from build123d import *

# Parameters (mm, degrees)
F0_R         = 10.3
F1_DEPTH     = 9
F3_R         = 3.1
F4_DEPTH     = 9.001
F6_DEPTH     = 1.8
F7_T4_ANGLE  = 359.64
F7_S5_R      = 3.1
F7_T6_DEPTH  = 5
F7_T10_ANGLE = 359.64
F7_S11_R     = 3.1
F7_T12_DEPTH = 5
F7_T16_ANGLE = 359.64
F7_S17_R     = 3.1
F7_T18_DEPTH = 5
F9_R         = 12.75
F10_DEPTH    = 25
F11_R        = 3.1
F12_DEPTH    = 34.0010001
F13_R        = 12.75
F13_R_2      = 11.35
F14_DEPTH    = 20
F16_DEPTH    = 5
F17_R        = 10.3
F18_DEPTH    = 34.0010001
F20_START    = -5
F20_DEPTH    = 5
F21_R        = 10.3
F21_R_2      = 9.3
F22_DEPTH    = 8
F23_R        = 0.99999


# Not quite as in the source:
# - a fillet or chamfer that OpenCascade refuses, or shapes differently, is made with other operations: its cross-section is extruded or revolved along the edge and cut away or added
# - a fillet or chamfer is up to 0.001 mm smaller than in the source, because OpenCascade refuses the exact size


with BuildPart() as f1:
    # F0 (on Front) → F1 (new body)
    with BuildSketch(Plane.XZ):
        Circle(F0_R)
    extrude(amount=F1_DEPTH)

    # F3 (on face) → F4 (cut, through all)
    with BuildSketch(Plane.XZ.offset(9)):
        Circle(F3_R)
    extrude(amount=-F4_DEPTH, mode=Mode.SUBTRACT)

    # F5 (on face) → F6 (cut)
    with BuildSketch(Plane.XZ.offset(9)):
        with BuildLine():
            ThreePointArc((-3.0819681678, 0.333874546), (-2.6846787517, 1.55), (-1.8301279224, 2.502125454))
            ThreePointArc((-1.8301279224, 2.502125454), (-6.4951905284, 3.75), (-3.0819681678, 0.333874546))
        make_face()
        with BuildLine():
            ThreePointArc((6.8301270189, 2.5), (4.331189746, 4.9999997741), (1.8301279224, 2.502125454))
            ThreePointArc((1.8301279224, 2.502125454), (2.6846787517, 1.55), (3.0819681678, 0.333874546))
            ThreePointArc((3.0819681678, 0.333874546), (5.5810472546, 0.3354680497), (6.8301270189, 2.5))
        make_face()
        with BuildLine():
            ThreePointArc((1.2518402454, -2.836), (0, -3.1), (-1.2518402454, -2.836))
            ThreePointArc((-1.2518402454, -2.836), (-1.2490795384, -7.1655946774), (2.5, -5))
            ThreePointArc((2.5, -5), (2.1655946774, -3.7509204616), (1.2518402454, -2.836))
        make_face()
    extrude(amount=-F6_DEPTH, mode=Mode.SUBTRACT)

    # F7: fillet of radius 1 on 3 edges, made by hand


with BuildPart() as f7_tool2:
    # F7_s3 → F7_t4 (revolve)
    with BuildSketch(Plane(origin=(0.0078111935, 0, 0.0136280797), x_dir=(0, 1, 0), z_dir=(-0.497276838, 0, -0.8675919239))):
        with BuildLine():
            ThreePointArc((-8.2, -2.499975326), (-7.4928932188, -2.7928685448), (-7.2, -3.499975326))
            Line((-7.2, -3.499975326), (-7.18, -3.499975326))
            Line((-7.18, -3.499975326), (-7.18, -2.479975326))
            Line((-7.18, -2.479975326), (-8.2, -2.479975326))
            Line((-8.2, -2.479975326), (-8.2, -2.499975326))
        make_face()
    revolve(axis=Axis((-4.3301270189, -7.2, 2.5), (0, -1, 0)), revolution_arc=F7_T4_ANGLE)

    # F7_s5 → F7_t6 (cut, symmetric)
    with BuildSketch(Plane.XZ.offset(7.7)):
        Circle(F7_S5_R)
    extrude(amount=F7_T6_DEPTH, both=True, mode=Mode.SUBTRACT)


with BuildPart() as f1_1:
    add(f1.part)

    # F7_t1: union F7_tool2
    add(f7_tool2.part)


with BuildPart() as f7_tool8:
    # F7_s9 → F7_t10 (revolve)
    with BuildSketch(Plane(origin=(0.0078966665, 0, -0.0135787318), x_dir=(0, 1, 0), z_dir=(-0.5027182272, 0, 0.8644503364))):
        with BuildLine():
            ThreePointArc((-8.2, -2.499975326), (-7.4928932188, -2.7928685448), (-7.2, -3.499975326))
            Line((-7.2, -3.499975326), (-7.18, -3.499975326))
            Line((-7.18, -3.499975326), (-7.18, -2.479975326))
            Line((-7.18, -2.479975326), (-8.2, -2.479975326))
            Line((-8.2, -2.479975326), (-8.2, -2.499975326))
        make_face()
    revolve(axis=Axis((4.3301270189, -7.2, 2.5), (0, -1, 0)), revolution_arc=F7_T10_ANGLE)

    # F7_s11 → F7_t12 (cut, symmetric)
    with BuildSketch(Plane.XZ.offset(7.7)):
        Circle(F7_S11_R)
    extrude(amount=F7_T12_DEPTH, both=True, mode=Mode.SUBTRACT)


with BuildPart() as f1_2:
    add(f1_1.part)

    # F7_t7: union F7_tool8
    add(f7_tool8.part)


with BuildPart() as f7_tool14:
    # F7_s15 → F7_t16 (revolve)
    with BuildSketch(Plane(origin=(-0.0157078599, 0, -4.93479e-05), x_dir=(0, 1, 0), z_dir=(0.9999950652, 0, 0.0031415875))):
        with BuildLine():
            ThreePointArc((-8.2, -2.499975326), (-7.4928932188, -2.7928685448), (-7.2, -3.499975326))
            Line((-7.2, -3.499975326), (-7.18, -3.499975326))
            Line((-7.18, -3.499975326), (-7.18, -2.479975326))
            Line((-7.18, -2.479975326), (-8.2, -2.479975326))
            Line((-8.2, -2.479975326), (-8.2, -2.499975326))
        make_face()
    revolve(axis=Axis((0, -7.2, -5), (0, -1, 0)), revolution_arc=F7_T16_ANGLE)

    # F7_s17 → F7_t18 (cut, symmetric)
    with BuildSketch(Plane.XZ.offset(7.7)):
        Circle(F7_S17_R)
    extrude(amount=F7_T18_DEPTH, both=True, mode=Mode.SUBTRACT)


with BuildPart() as f1_3:
    add(f1_2.part)

    # F7_t13: union F7_tool14
    add(f7_tool14.part)

    # F9 (on offset) → F10 (join)
    with BuildSketch(Plane(origin=(0, 0, 0), x_dir=(-1, 0, 0), z_dir=(0, 1, 0))):
        Circle(F9_R)
    extrude(amount=F10_DEPTH)

    # F11 (on face) → F12 (cut, through all)
    with BuildSketch(Plane(origin=(0, 25, 0), x_dir=(-1, 0, 0), z_dir=(0, 1, 0))):
        Circle(F11_R)
    extrude(amount=-F12_DEPTH, mode=Mode.SUBTRACT)

    # F13 (on face) → F14 (cut)
    with BuildSketch(Plane(origin=(0, 25, 0), x_dir=(-1, 0, 0), z_dir=(0, 1, 0))):
        Circle(F13_R)
        Circle(F13_R_2, mode=Mode.SUBTRACT)
    extrude(amount=-F14_DEPTH, mode=Mode.SUBTRACT)

    # F15 (on face) → F16 (join)
    with BuildSketch(Plane(origin=(0, 5, 0), x_dir=(-1, 0, 0), z_dir=(0, 1, 0))):
        with BuildLine():
            ThreePointArc((2, 12.5921602595), (0, 12.75), (-2, 12.5921602595))
            Line((-2, 12.5921602595), (-2, 11.1723990262))
            ThreePointArc((-2, 11.1723990262), (0, 11.35), (2, 11.1723990262))
            Line((2, 11.1723990262), (2, 12.5921602595))
        make_face()
        with BuildLine():
            ThreePointArc((2, -11.1723990262), (0, -11.35), (-2, -11.1723990262))
            Line((-2, -11.1723990262), (-2, -12.5921602595))
            ThreePointArc((-2, -12.5921602595), (0, -12.75), (2, -12.5921602595))
            Line((2, -12.5921602595), (2, -11.1723990262))
        make_face()
    extrude(amount=F16_DEPTH)

    # F17 (on face) → F18 (cut, through all)
    with BuildSketch(Plane.XZ.offset(9)):
        Circle(F17_R)
    extrude(amount=-F18_DEPTH, mode=Mode.SUBTRACT)

    # F19 (on face) → F20 (join)
    with BuildSketch(Plane(origin=(0, 25, 0), x_dir=(-1, 0, 0), z_dir=(0, 1, 0)).offset(F20_START)):
        with BuildLine():
            Line((-7.5, 0), (-10.3, 0))
            ThreePointArc((-10.3, 0), (-9.5744451536, -3.7973675092), (-7.5, -7.0597450379))
            Line((-7.5, -7.0597450379), (-7.5, 0))
        make_face()
    extrude(amount=-F20_DEPTH)

    # F21 (on face) → F22 (join)
    with BuildSketch(Plane.XZ.offset(-15)):
        Circle(F21_R)
        Circle(F21_R_2, mode=Mode.SUBTRACT)
    extrude(amount=F22_DEPTH)

    # F23 (radius 1 in the source; OpenCascade refuses exactly that, so slightly less here)
    f23_edges = [f1_3.edges().sort_by_distance(p)[0] for p in [
        (-9.3, 7, 0),
    ]]
    fillet(f23_edges, radius=F23_R)


solid = f1_3.part
Model file for the job. Use its own axes, mm. A direction names the side the tool comes from. Give positions to 0.01 mm unless a question says otherwise; leave off trailing zeros. Write each loop counter-clockwise with the first axis right and the second up, starting at its lowest first coordinate (ties: lowest second). Pieces come first, ordered by that corner, then holes. Notation, with made-up numbers: (-1.5, 48) -> (34.5, 48) arc R25 cw to (34.5, 70) -> close; hole circle Ø3 at (61.25, 74). An arc over 180 degrees is marked (long way). Write item = value, one per line.
(1) Tool access for faces 3 (the face through (-12, 5, 0)), 4 (the face through (2, 7, -12)), 5 (the face through (-9.2, 15, 2.3)): list every direction of +Z, -Z, +X, -X, +Y, -Y with a clear straight run to the whole face (end or side of a thin tool).
Determined:
face_3 = -X, +Y
face_4 = -Z, +X, +Y
face_5 = +Y
(2) Probe line 1 along Z through (x, y) = (0, 10.75); line 2 along X through (y, z) = (20.75, 0); line 3 along Z through (x, y) = (0, 9.5). List the from-to ranges inside material, lowest first.
Determined:
line_1 = -11.35 to -9.3, 9.3 to 11.35
line_2 = -11.35 to -10.3, 10.3 to 11.35
line_3 = -12.75 to -9.3, 9.3 to 12.75
(3) Flat gauge pins, fed straight in: P1, Ø1.4, axis at x = 8.5, y = 18.5, coming from the +Z side; P2, Ø1.4, axis at x = 8.5, z = -3.5, coming from the -Y side; P3, Ø1.1, axis at y = 7, z = -12, coming from the -X side; P4, Ø5.5, axis at x = -7, z = 5.5, coming from the +Y side. Where does each tip first touch, or does it go through?
Determined:
P1 = 8.25
P2 = 7.09
P3 = -2
P4 = 25
(4) Slice it at C-C, the plane y = 11. Give the cut face in (x, z).
Determined:
outline = circle Ø22.7 at (0, 0); hole circle Ø18.6 at (0, 0)
(5) Mould opens along Z. For faces 1 (the face through (0, 10, -12)), 2 (the face through (9, 18, 0)) say: released by +Z, released by -Z, zero draft, split by the parting line, or undercut.
Determined:
face_1 = zero draft
face_2 = undercut
(6) Slice it at B-B, the plane y = 7.5. Give the cut face in (x, z), then the cut area to 3 significant figures.
Determined:
outline = (-2, -12.59) arc R12.75 ccw to (2, -12.59) -> (2, -11.17) arc R11.35 ccw to (2, 11.17) -> (2, 12.59) arc R12.75 ccw to (-2, 12.59) -> (-2, 11.17) arc R11.35 ccw to (-2, -11.17) -> close; hole circle Ø18.87 at (0, 0)
area = 136 mm2
